```python
from build123d import *

# Parameters (mm, degrees)
ARRAY_X_COUNT    = 3
ARRAY_X_PITCH    = 8.485281
ARRAY001_X_COUNT = 2
ARRAY001_X_PITCH = 12
ARRAY001_Y_COUNT = 2
ARRAY001_Y_PITCH = 12
BOX001_W         = 16
BOX001_H         = 1
BOX001_DEPTH     = 4
BOX_W            = 20
BOX_H            = 40
BOX_DEPTH        = 10


with BuildPart() as numero3:
    # Sphere → Sphere (revolve)
    with BuildSketch(Plane(origin=(4, 37, 10), x_dir=(1, 0, 0), z_dir=(0, -1, 0))):
        with BuildLine():
            ThreePointArc((0, -2), (2, 0), (0, 2))
            Line((0, 2), (0, -2))
        make_face()
    revolve(axis=Axis((4, 37, 10), (0, 0, 1)))

    # Array X: numero3 ×3


with BuildPart() as numero3_1:
    add(numero3.part)
    with Locations(*[Vector(0.707107, -0.707107, 0) * (i * ARRAY_X_PITCH) for i in range(1, ARRAY_X_COUNT)]):
        add(numero3.part)


with BuildPart() as array001:
    # Sphere001 → Sphere001 (revolve)
    with BuildSketch(Plane.XZ):
        with BuildLine():
            ThreePointArc((0, -2), (2, 0), (0, 2))
            Line((0, 2), (0, -2))
        make_face()
    revolve(axis=Axis((0, 0, 0), (0, 0, 1)))

    # Array001 X: Array001 ×2


with BuildPart() as array001_1:
    add(array001.part)
    with Locations(*[(i * ARRAY001_X_PITCH, 0, 0) for i in range(1, ARRAY001_X_COUNT)]):
        add(array001.part)

    # Array001 Y: Array001 ×2


with BuildPart() as array001_2:
    add(array001_1.part)
    with Locations(*[(0, i * ARRAY001_Y_PITCH, 0) for i in range(1, ARRAY001_Y_COUNT)]):
        add(array001_1.part)


with BuildPart() as array001_3:
    # Array001 placement: moved
    add(array001_2.part.moved(Location((4, 4, 10))))


with BuildPart() as sphere002:
    # Sphere002 → Sphere002 (revolve)
    with BuildSketch(Plane(origin=(10, 10, 10), x_dir=(1, 0, 0), z_dir=(0, -1, 0))):
        with BuildLine():
            ThreePointArc((0, -2), (2, 0), (0, 2))
            Line((0, 2), (0, -2))
        make_face()
    revolve(axis=Axis((10, 10, 10), (0, 0, 1)))


with BuildPart() as cube:
    # Box001 → Box001 (new body)
    with BuildSketch(Plane(origin=(2, 20, 7), x_dir=(1, 0, 0), z_dir=(0, 0, 1))):
        with Locations((8, 0.5)):
            Rectangle(BOX001_W, BOX001_H)
    extrude(amount=BOX001_DEPTH)


with BuildPart() as cut003:
    # Box → Box (new body)
    with BuildSketch(Plane.XY):
        with Locations((10, 20)):
            Rectangle(BOX_W, BOX_H)
    extrude(amount=BOX_DEPTH)

    # Cut: cut Cube
    add(cube.part, mode=Mode.SUBTRACT)

    # Cut001: cut Sphere002
    add(sphere002.part, mode=Mode.SUBTRACT)

    # Cut002: cut Array001
    add(array001_3.part, mode=Mode.SUBTRACT)

    # Cut003: cut numero3
    add(numero3_1.part, mode=Mode.SUBTRACT)


solid = cut003.part
```
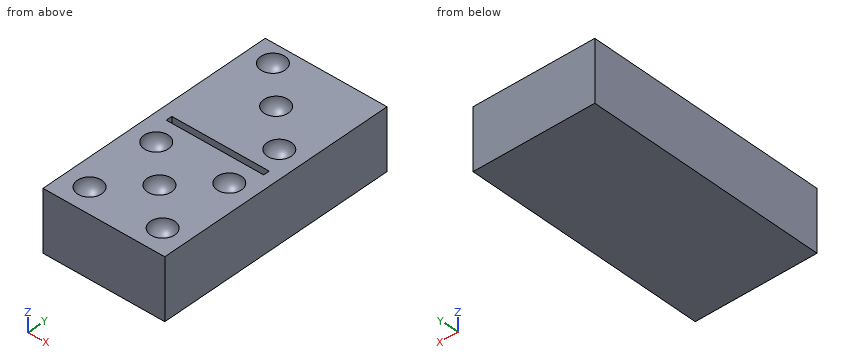
Verification items for the finished model (mm, model axes). Give positions to 0.01 mm unless a question says otherwise; leave off trailing zeros. Order: outer loops, then holes, each group sorted by start corner. A loop starts at its lowest first (then second) coordinate and runs counter-clockwise, first axis right, second up. Notation, with made-up numbers: (60, -14.75) -> (80, -14.75) arc R27 cw to (80, 10.25) -> close; hole circle Ø11 at (-11, 69). An arc over 180 degrees is marked (long way). Use a Markdown table: item, result.
1) Material ranges on probe 1 along X at (y, z) = (3, 9.25); probe 2 along Y at (x, z) = (3.75, 9.5); probe 3 along Y at (x, z) = (2.75, 7.25), recorded low to high.
Results:
| item | result |
|---|---|
| probe 1 | 0 to 2.44, 5.56 to 14.44, 17.56 to 20 |
| probe 2 | 0 to 2.08, 5.92 to 14.08, 17.92 to 20, 21 to 35.08, 38.92 to 40 |
| probe 3 | 0 to 20, 21 to 40 |
2) Section check A-A, the plane z = 9. Give the number of separate pieces and of enclosed holes in the cut face, then the cut area to 3 significant figures.
Results:
| item | result |
|---|---|
| separate pieces | 1 |
| enclosed holes | 9 |
| area | 709 mm² |
3) Section check C-C, the plane y = 32. Record the boundary of the cut face in (x, z), then the cut area to 3 significant figures.
Results:
| item | result |
|---|---|
| outline | (0, 0) -> (20, 0) -> (20, 10) -> (11.73, 10) arc R1.73 cw to (8.27, 10) -> (0, 10) -> close |
| area | 195 mm² |
4) Section check D-D, the plane x = 11. Record the boundary of the cut face in (y, z).
Results:
| item | result |
|---|---|
| outline | (0, 0) -> (40, 0) -> (40, 10) -> (32.73, 10) arc R1.73 cw to (29.27, 10) -> (21, 10) -> (21, 7) -> (20, 7) -> (20, 10) -> (11.73, 10) arc R1.73 cw to (8.27, 10) -> (0, 10) -> close |
5) Section check B-B, the plane x = 17.5. Record the boundary of the cut face in (y, z).
Results:
| item | result |
|---|---|
| outline | (0, 0) -> (40, 0) -> (40, 10) -> (26.32, 10) arc R1.32 cw to (23.68, 10) -> (21, 10) -> (21, 7) -> (20, 7) -> (20, 10) -> (17.32, 10) arc R1.32 cw to (14.68, 10) -> (5.32, 10) arc R1.32 cw to (2.68, 10) -> (0, 10) -> close |
